Check sheet for the modelled part. Datum: model origin and axes. Units: mm. A direction names the side the tool comes from. Give positions to 0.01 mm unless a question says otherwise; leave off trailing zeros. Loops run counter-clockwise (first coordinate to the right, second up) from the corner with the lowest first, then second, coordinate; pieces in that order, holes last. Notation, with made-up numbers: (31.25, 72.25) -> (87.25, 72.25) arc R24 cw to (87.25, 111.25) -> close; hole circle Ø9 at (46.25, -28). An arc over 180 degrees is marked (long way). Write each question's results on one line, items separated by ' | '. Start each with the question number.
1. Material ranges on L1, parallel to Z at x = 0, y = 2.8; L2, parallel to Z at x = 0, y = -0.25; L3, parallel to X at y = -3.5, z = 2.5, recorded low to high. Write a range as from..to.
2. Gauge pin test, flat ends, axial feed: pin 1 Ø2 at (y, z) = (3, 35) entering from -X; pin 2 Ø5 at (x, z) = (-18, -21) entering from -Y; pin 3 Ø4 at (y, z) = (-0.5, -13.5) entering from -X. Record the tip position at first contact, or that the pin passes through.
3. Cross-section at D-D on x = -18. Record the boundary of the cut face in (y, z), and give its area (3 significant figures).
4. Cross-section at A-A on x = 0. Record the boundary of the cut face in (y, z).
5. Mould release check, pull along X, two halves, no side actions. Record for faces 1 (the face through (47.69, -0.1, 15.02)), 2 (the face through (-28, -4, -21)), 3 (the face through (6.5, -7, -3.1)): +X half, -X half, draft (parallel to the pull), parting line (faces both ways), or undercut.
6. Tool access check on faces 4 (the face through (-34, 7, -10)), 5 (the face through (15, 1.5, -7)), 6 (the face through (15, -1.5, -7)). Record the directions out of +Z, -Z, +X, -X, +Y, -Y that give a thin tool (end or side, any length) a straight path to the whole face; none if there is none.
7. Cross-section at B-B on z = 0. Record the boundary of the cut face in (x, y), and give its area (3 significant figures).
8. Cross-section at C-C on y = -5.5. Record the boundary of the cut face in (x, z).
from build123d import *

# Parameters (mm, degrees)
F0_R     = 35
F0_R_2   = 15
F1_DEPTH = 1.5
F1_TAPER = -3
F0_R_3   = 50
F2_DEPTH = 7
F0_R_4   = 7
F3_DEPTH = 7


with BuildPart() as f1:
    # F0 (on Front) → F1 (new body, symmetric)
    with BuildSketch(Plane.XZ):
        Circle(F0_R)
        Circle(F0_R_2, mode=Mode.SUBTRACT)
    extrude(amount=F1_DEPTH, both=True, taper=F1_TAPER)

    # F0 (on Front) → F2 (join, symmetric)
    with BuildSketch(Plane.XZ):
        Circle(F0_R_3)
        Circle(F0_R, mode=Mode.SUBTRACT)
    extrude(amount=F2_DEPTH, both=True)

    # F0 (on Front) → F3 (join, symmetric)
    with BuildSketch(Plane.XZ):
        Circle(F0_R_2)
        Circle(F0_R_4, mode=Mode.SUBTRACT)
    extrude(amount=F3_DEPTH, both=True)


solid = f1.part
Geometry says:
1) L1: -50..-35, -15..-7, 7..15, 35..50 | L2: -50..-7, 7..50 | L3: -49.94..-34.91, -14.79..-6.54, 6.54..14.79, 34.91..49.94
2) pin 1: x = -36.66 | pin 2: y = -1.5 | pin 3: x = -48.66
3) outline: (-7, -46.65) -> (7, -46.65) -> (7, -30.02) -> (1.5, -30.02) -> (1.5, 30.02) -> (7, 30.02) -> (7, 46.65) -> (-7, 46.65) -> (-7, 30.02) -> (-1.5, 30.02) -> (-1.5, -30.02) -> (-7, -30.02) -> close | area: 646 mm^2
4) outline: (-7, -50) -> (7, -50) -> (7, -35) -> (1.5, -35) -> (1.5, -15) -> (7, -15) -> (7, -7) -> (-7, -7) -> (-7, -15) -> (-1.5, -15) -> (-1.5, -35) -> (-7, -35) -> close; (-7, 7) -> (7, 7) -> (7, 15) -> (1.5, 15) -> (1.5, 35) -> (7, 35) -> (7, 50) -> (-7, 50) -> (-7, 35) -> (-1.5, 35) -> (-1.5, 15) -> (-7, 15) -> close
5) face 1: parting line | face 2: undercut | face 3: draft
6) face 4: +Z, -Z, +X, -X, +Y | face 5: +Y | face 6: -Y
7) outline: (-50, -7) -> (-35, -7) -> (-35, -1.5) -> (-15, -1.5) -> (-15, -7) -> (-7, -7) -> (-7, 7) -> (-15, 7) -> (-15, 1.5) -> (-35, 1.5) -> (-35, 7) -> (-50, 7) -> close; (7, -7) -> (15, -7) -> (15, -1.5) -> (35, -1.5) -> (35, -7) -> (50, -7) -> (50, 7) -> (35, 7) -> (35, 1.5) -> (15, 1.5) -> (15, 7) -> (7, 7) -> close | area: 764 mm^2
8) outline: circle Ø100 at (0, 0); circle Ø30 at (0, 0); hole circle Ø70 at (0, 0); hole circle Ø14 at (0, 0)
